Solid Edge part; units mm, degrees
sketch "Sketch1" plane through (0, 0, 0) normal (0, -1, 0) x (1, 0, 0)
  line L0 (140, 0) -> (140, 35)
  line L1 (140, 35) -> (120, 35)
  line L2 (120, 35) -> (120, 65)
  line L3 (120, 65) -> (100, 65)
  line L4 (100, 65) -> (100, 40)
  line L5 (40, 40) -> (100, 40)
  line L6 (40, 65) -> (40, 40)
  line L7 (20, 65) -> (40, 65)
  line L8 (20, 35) -> (20, 65)
  line L9 (0, 35) -> (20, 35)
  line L10 (0, 35) -> (0, 0)
  line L11 (140, 0) -> (0, 0)
extrude "Protrusion1" add sketch "Sketch1" against normal blind 70
sketch "Sketch2" plane through (120, 35, 50) normal (1, 0, 0) x (0, 1, 0)
  circle A0 centre (0, 15) radius 20
extrude "ExtrudedCutout_1" cut sketch "Sketch2" against normal blind 180.6982
sketch "Sketch3" plane through (130, 35, 35) normal (0, 0, 1) x (1, 0, 0)
  circle A0 centre (-1.6363, 0) radius 5
  circle A1 centre (-120, 0) radius 5
extrude "ExtrudedCutout_2" cut sketch "Sketch3" against normal blind 2.3183
Geometry: final body of the model. Coordinates: model frame, mm. A direction names the side the tool comes from. Coordinates: 2 decimals unless noted, no trailing zeros. Loops run counter-clockwise (first coordinate to the right, second up) from the corner with the lowest first, then second, coordinate; pieces in that order, holes last. Notation, with made-up numbers: (82, -23.75) - (127, -23.75) arc R23 ccw to (127, 4.25) - close; hole circle Ø4 at (55, 32). An arc over 180 degrees is marked (long way). One line per question, with ' | ' between items. Start each with the question number.
(1) First-contact query: pin 1 (8 mm diameter, centred on y = 34, z = 52, fed in from -X); pin 2 (2 mm diameter, centred on x = 120.5, y = 26.5, fed in from -Z); pin 3 (6 mm diameter, centred on x = 10, y = 28.5, fed in from +Z); pin 4 (12.5 mm diameter, centred on y = 23, z = 51.5, fed in from +X). Flat tips, straight axial feed; report the tip coordinate or a pass-through.
(2) Reachability of faces 4 (the flat face through (70, 35, 40)), 5 (the flat face through (135, 35, 35)), 6 (the flat face through (71, 0, 26)), 7 (the flat face through (10, 35, 32.682)) from +Z, -Z, +X, -X, +Y, -Y: full face, straight path, thin tool, end or side. Return the list, or none.
(3) Cut plane D-D on y = 66.5. Output: boundary loops of the cut face in (x, z), and give its area (3 significant figures).
(4) Cut plane A-A on y = 35. Output: boundary loops of the cut face in (x, z), and give its area (3 significant figures).
(5) Cut plane C-C on x = 10. Output: boundary loops of the cut face in (y, z), and give its area (3 significant figures).
(6) Cut plane B-B on z = 56. Output: boundary loops of the cut face in (x, y), and give its area (3 significant figures).
(7) Ray query, L1, parallel to X at y = 20, z = 48; L2, parallel to Y at x = 10, z = 34.55; L3, parallel to Z at x = 93.5, y = 33.5. Return the intervals inside material, ascending. Write a range as from..to.
(8) Draft query along X for faces 1 (the flat face through (30, 62, 65)), 2 (the flat face through (100, 35, 44)), 3 (the flat face through (140, 35, 17)). Return one class per face: +X half, -X half, draft (parallel to the pull), parting line (faces both ways), or undercut.
Here are the results:
1) pin 1: through | pin 2: z = 0 | pin 3: z = 35 | pin 4: x = 120
2) face 4: +Z, +Y, -Y | face 5: +Z, +X, +Y, -Y | face 6: +Z, -Z, +X, -X, -Y | face 7: +Z
3) outline: (0, 0) - (140, 0) - (140, 35) - (120, 35) - (120, 65) - (100, 65) - (100, 40) - (40, 40) - (40, 65) - (20, 65) - (20, 35) - (0, 35) - close | area: 6,400 mm²
4) outline: (0, 0) - (140, 0) - (140, 35) - (133.36, 35) - (133.36, 32.68) - (123.36, 32.68) - (123.36, 35) - (120, 35) - (120, 45) - (100, 45) - (100, 40) - (40, 40) - (40, 45) - (20, 45) - (20, 35) - (15, 35) - (15, 32.68) - (5, 32.68) - (5, 35) - (0, 35) - close | area: 5,550 mm²
5) outline: (0, 0) - (70, 0) - (70, 35) - (40, 35) - (40, 32.68) - (30, 32.68) - (30, 35) - (0, 35) - close | area: 2,430 mm²
6) outline: (20, 0) - (40, 0) - (40, 17.14) - (20, 17.14) - close; (20, 52.86) - (40, 52.86) - (40, 70) - (20, 70) - close; (100, 0) - (120, 0) - (120, 17.14) - (100, 17.14) - close; (100, 52.86) - (120, 52.86) - (120, 70) - (100, 70) - close | area: 1,370 mm²
7) L1: 20..40, 100..120 | L2: 0..30, 40..70 | L3: 0..40
8) face 1: draft | face 2: undercut | face 3: +X half
